```python
from build123d import *

# Parameters (mm, degrees)
SKETCH1_R           = 3
SKETCH1_R_2         = 2.7
BOSS_EXTRUDE1_DEPTH = 5
FILLET1_R           = 10


with BuildPart() as part:
    # Sketch1 → Boss-Extrude1 (new body)
    with BuildSketch(Plane.XY):
        Polygon((-25, 22), (-25, 70), (-80, 70), (-80, 65), (-85, 65), (-85, 60), (-80, 60), (-80, 56.5), (-77, 56.5), (-77, 57.6), (-74.7, 57.6), (-74.7, 56.5), (-70, 56.5), (-70, 53.5), (-74.7, 53.5), (-74.7, 52.4), (-77, 52.4), (-77, 53.5), (-80, 53.5), (-80, 50), (-85, 50), (-85, 45), (-80, 45), (-80, 25), (-85, 25), (-85, 20), (-80, 20), (-80, 16.5), (-77, 16.5), (-77, 17.6), (-74.7, 17.6), (-74.7, 16.5), (-70, 16.5), (-70, 13.5), (-74.7, 13.5), (-74.7, 12.4), (-77, 12.4), (-77, 13.5), (-80, 13.5), (-80, 10), (-85, 10), (-85, 5), (-80, 5), (-80, 0), (-72, 0), align=None)
        with Locations((-65.5, 29.5)):
            Circle(SKETCH1_R, mode=Mode.SUBTRACT)
        with Locations((-34.5, 29.5)):
            Circle(SKETCH1_R, mode=Mode.SUBTRACT)
        with Locations((-50, 45)):
            Circle(SKETCH1_R_2, mode=Mode.SUBTRACT)
        with Locations((-65.5, 60.5)):
            Circle(SKETCH1_R, mode=Mode.SUBTRACT)
        with Locations((-34.5, 60.5)):
            Circle(SKETCH1_R, mode=Mode.SUBTRACT)
    extrude(amount=BOSS_EXTRUDE1_DEPTH)

    # Fillet1
    fillet1_edges = [part.edges().sort_by_distance(p)[0] for p in [
        (-72, 0, 2.5),
        (-25, 70, 2.5),
        (-25, 22, 2.5),
    ]]
    fillet(fillet1_edges, radius=FILLET1_R)


solid = part.part
```
Can you work these out from the model? Positions are in its coordinate system, mm. A direction names the side the tool comes from. Round coordinates to 2 decimals unless told otherwise and drop trailing zeros. Loops run counter-clockwise (first coordinate to the right, second up) from the corner with the lowest first, then second, coordinate; pieces in that order, holes last. Notation, with made-up numbers: M -24.5,-10 L -12.5,-10 A22 cw -12.5,13 Z; hole C -20,1 d11. An arc over 180 degrees is marked long. Write item = value, one per line. Start each with the question number.
(1) Suppose I cut it at C-C on z = 1.1. Give the number of separate pieces and of enclosed holes in the cut face, plus the area to 3 significant figures.
(2) If we mould it in two halves opening along Y, with no side actions, what happens to faces 1 (the face through (-82, 65, 2)), 2 (the face through (-79, 16.5, 2)), 3 (the face through (-72.023, 0.245, 2.535))? For each: released by +Y, released by -Y, zero draft, split by the parting line, or undercut.
(3) Which directions (+Z, -Z, +X, -X, +Y, -Y) give clear straight access to the entire face, cutting with the end or side of a thin tool? Please do faces 4 (the face through (-82, 25, 2)), 5 (the face through (-76, 12.4, 2)), 6 (the face through (-85, 48, 2)).
(4) I need wall thicknesses on line 1 along Y through (x, z) = (-76.5, 1.25); line 2 along Y through (x, z) = (-79.5, 2.15); line 3 along X through (y, z) = (31, 3.9). Which ranges of each line are inside material? Lowest first, please.
(5) Suppose I cut it at D-D on x = -65.5. Write out the boundary of the cut face in (y, z).
(6) Suppose I cut it at B-B on x = -34. Write out the boundary of the cut face in (y, z).
(7) Suppose I cut it at A-A on x = -50. Write out the boundary of the cut face in (y, z).
(8) I'm going to push flat-ended pins straight in: P1, Ø2.5, axis at y = 66.5, z = 3, coming from the -X side; P2, Ø0.9, axis at y = 55.5, z = 1.5, coming from the -X side; P3, Ø3.5, axis at x = -65.5, y = 29.5, coming from the -Z side. Where does each tip first touch, or does it pass through?
Answer block:
q1.separate_pieces = 1
q1.enclosed_holes = 5
q1.area = 3,200 mm²
q2.face_1 = released by +Y
q2.face_2 = undercut
q2.face_3 = released by -Y
q3.face_4 = +Z, -Z, -X
q3.face_5 = +Z, -Z
q3.face_6 = +Z, -Z, -X, +Y, -Y
q4.line_1 = 0 to 12.4, 17.6 to 52.4, 57.6 to 70
q4.line_2 = 0 to 13.5, 16.5 to 53.5, 56.5 to 70
q4.line_3 = -80 to -68.1, -62.9 to -37.1, -31.9 to -25
q5.outline = M 3.04,0 L 26.5,0 L 26.5,5 L 3.04,5 Z; M 32.5,0 L 57.5,0 L 57.5,5 L 32.5,5 Z; M 63.5,0 L 70,0 L 70,5 L 63.5,5 Z
q6.outline = M 17.79,0 L 26.54,0 L 26.54,5 L 17.79,5 Z; M 32.46,0 L 57.54,0 L 57.54,5 L 32.46,5 Z; M 63.46,0 L 69.95,0 L 69.95,5 L 63.46,5 Z
q7.outline = M 10.3,0 L 42.3,0 L 42.3,5 L 10.3,5 Z; M 47.7,0 L 70,0 L 70,5 L 47.7,5 Z
q8.P1 = -80
q8.P2 = -70
q8.P3 = through
